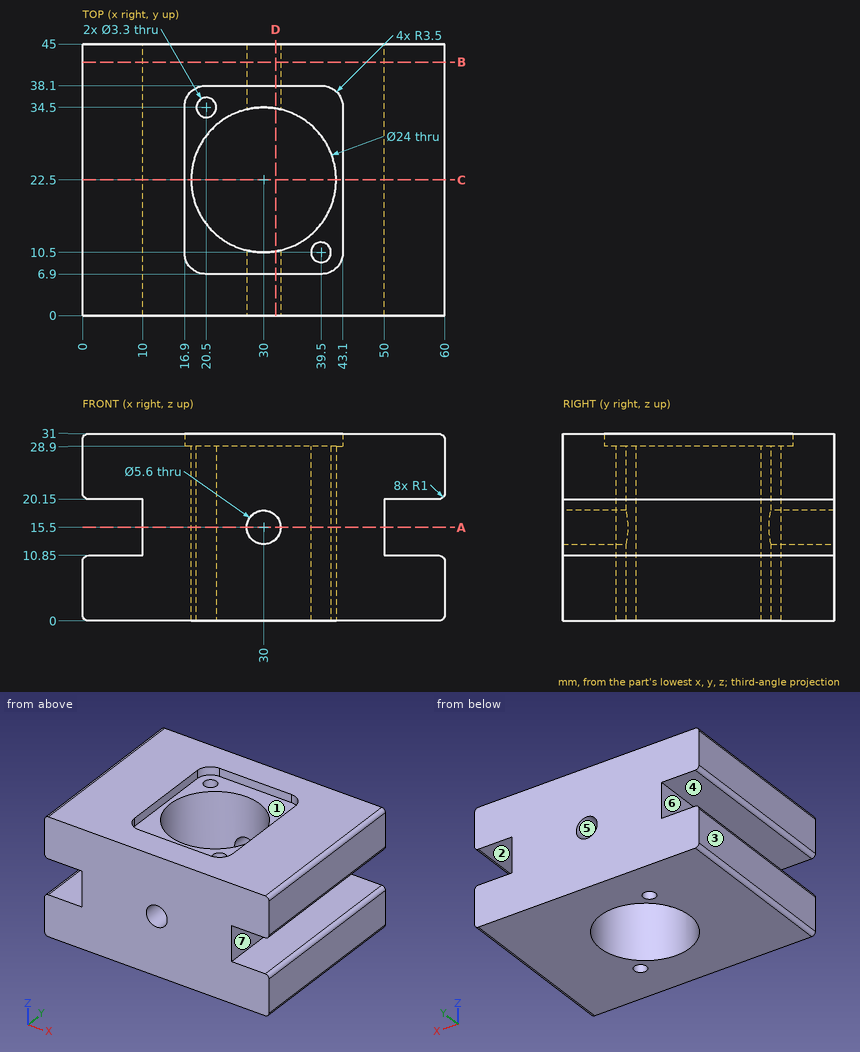
For this review, use the dimensioned drawing (mm, ordinates from the lowest corner) and the shaded views. A direction names the side the tool comes from. Coordinates: 2 decimals unless noted, no trailing zeros. Order: outer loops, then holes, each group sorted by start corner. A loop starts at its lowest first (then second) coordinate and runs counter-clockwise, first axis right, second up. Notation, with made-up numbers: M 73.25,-35 L 129.25,-35 A29 ccw 129.25,0 Z; hole C 5.5,-17 d3. An arc over 180 degrees is marked long. Answer as a JSON object with one key per item and string values. Group by question number.
1) Add section C-C, the plane y = 22.5. Write out the cut boundary in (x, z).
2) Wall thickness on L1, parallel to X at y = 3.5, z = 15.5; L2, parallel to Z at x = 51.5, y = 15.5; L3, parallel to Y at x = 20.5, z = 22.25: over which ranges is each line inside the solid? List them lowest first.
3) For pin 1 (3 mm diameter, centred on y = 17, z = 17, fed in from +X); pin 2 (21 mm diameter, centred on x = 32, y = 24, fed in from +Z); pin 3 (4.5 mm diameter, centred on y = 33.5, z = 16.5, fed in from -X), all flat-tipped, find the tip position at first contact; note any pin that passes through.
4) Add section D-D, the plane x = 32. Write out the cut boundary in (y, z).
5) Tool access review of the marked faces 5, 6 and 7: name each direction out of +Z, -Z, +X, -X, +Y, -Y from which nothing blocks a thin tool from reaching the whole face with its end or side.
6) Add section B-B, the plane y = 42. Write out the cut boundary in (x, z).
7) Mouldability with a two-part tool opening along Z and no side actions: class the marked faces 1, 2, 3 and 4 as pulls with the +Z half, pulls with the -Z half, needs draft (parallel to the pull), parting line crosses it, or undercut.
8) Add section A-A, the plane z = 15.5. Write out the cut boundary in (x, y), then the cut area to 3 significant figures.
Computed values:
{
 "1": {"outline": "M 0,1 A1 ccw 1,0 L 18,0 L 18,28.9 L 16.9,28.9 L 16.9,31 L 1,31 A1 ccw 0,30 L 0,21.15 A1 ccw 1,20.15 L 10,20.15 L 10,10.85 L 1,10.85 A1 ccw 0,9.85 Z; M 42,0 L 59,0 A1 ccw 60,1 L 60,9.85 A1 ccw 59,10.85 L 50,10.85 L 50,20.15 L 59,20.15 A1 ccw 60,21.15 L 60,30 A1 ccw 59,31 L 43.1,31 L 43.1,28.9 L 42,28.9 Z"},
 "2": {"L1": "x = 10 to 27.2, 32.8 to 50", "L2": "z = 0 to 10.85, 20.15 to 31", "L3": "y = 0 to 15.17, 29.83 to 32.85, 36.15 to 45"},
 "3": {"pin 1": "stops at x = 50", "pin 2": "stops at z = 28.9", "pin 3": "stops at x = 10"},
 "4": {"outline": "M 0,0 L 10.67,0 L 10.67,13.54 L 0,13.54 Z; M 0,17.46 L 10.67,17.46 L 10.67,28.9 L 6.9,28.9 L 6.9,31 L 0,31 Z; M 34.33,0 L 45,0 L 45,13.54 L 34.33,13.54 Z; M 34.33,17.46 L 45,17.46 L 45,31 L 38.1,31 L 38.1,28.9 L 34.33,28.9 Z"},
 "5": {"face 5": "+Y, -Y", "face 6": "-X, +Y, -Y", "face 7": "+X, +Y, -Y"},
 "6": {"outline": "M 0,1 A1 ccw 1,0 L 59,0 A1 ccw 60,1 L 60,9.85 A1 ccw 59,10.85 L 50,10.85 L 50,20.15 L 59,20.15 A1 ccw 60,21.15 L 60,30 A1 ccw 59,31 L 1,31 A1 ccw 0,30 L 0,21.15 A1 ccw 1,20.15 L 10,20.15 L 10,10.85 L 1,10.85 A1 ccw 0,9.85 Z; hole C 30,15.5 d5.6"},
 "7": {"face 1": "pulls with the +Z half", "face 2": "undercut", "face 3": "needs draft", "face 4": "undercut"},
 "8": {"outline": "M 10,0 L 27.2,0 L 27.2,10.83 A12 cw 27.2,34.17 L 27.2,45 L 10,45 Z; M 32.8,0 L 50,0 L 50,45 L 32.8,45 L 32.8,34.17 A12 cw 32.8,10.83 Z; hole C 20.5,34.5 d3.3; hole C 39.5,10.5 d3.3", "area": "1,210 mm^2"}
}
